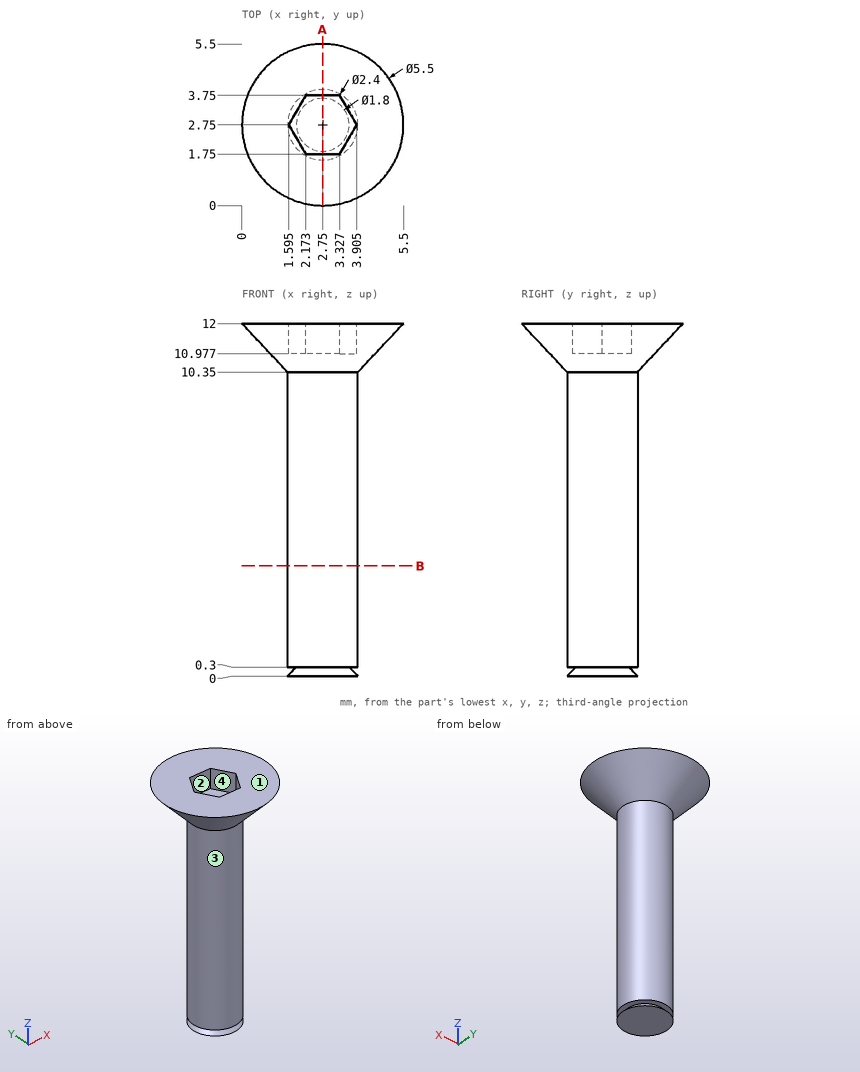
Geometry check sheet. Reference: drawing and pictorial views, mm from the part's lowest x, y, z. Give positions to 0.01 mm unless a question says otherwise; leave off trailing zeros. Write each loop counter-clockwise with the first axis right and the second up, starting at its lowest first coordinate (ties: lowest second). Pieces come first, ordered by that corner, then holes. Notation, with made-up numbers: (-12.75, 31.5) -> (5.25, 31.5) arc R22 cw to (5.25, 67.5) -> close; hole circle Ø1 at (-22, -38.5). An arc over 180 degrees is marked (long way). One line per item, written item: value. Start each with the question number.
Item 1: Material ranges on probe 1 along Z at (x, y) = (3.5, 2.6); probe 2 along Y at (x, z) = (2.8, 8.25); probe 3 along X at (y, z) = (3.1, 11.25) (1 decimal), recorded low to high. Write a range as from..to.
Item 2: Draft check along X on the marked faces 1, 2, 3 and 4. Enter one of: +X half, -X half, draft (parallel to the pull), parting line (faces both ways), or undercut.
Item 3: Section check B-B on z = 3.75. Record the cut outline in (x, y).
Item 4: Section check A-A on x = 2.75. Record the cut outline in (y, z).
Item 5: Gauge pin test, flat ends, axial feed: pin 1 (0.8 mm diameter, centred on x = 2.5, z = 11.5, fed in from +Y) (1 decimal); pin 2 (2 mm diameter, centred on x = 4.5, z = 4.5, fed in from +Y); pin 3 (0.7 mm diameter, centred on x = 2.5, y = 2.5, fed in from -Z); pin 4 (1 mm diameter, centred on x = 3, y = 2.5, fed in from +Z). Record the tip position at first contact, or that the pin passes through.
Results list:
1. probe 1: 0..10.98
1. probe 2: 1.55..3.95
1. probe 3: 0.7..1.8, 3.7..4.8
2. face 1: draft
2. face 2: undercut
2. face 3: parting line
2. face 4: undercut
3. outline: circle Ø2.4 at (2.75, 2.75)
4. outline: (0, 12) -> (1.55, 10.35) -> (1.55, 0.3) -> (1.85, 0.3) -> (1.55, 0) -> (3.95, 0) -> (3.65, 0.3) -> (3.95, 0.3) -> (3.95, 10.35) -> (5.5, 12) -> (3.75, 12) -> (3.75, 10.98) -> (1.75, 10.98) -> (1.75, 12) -> close
5. pin 1: y = 5.4
5. pin 2: y = 3.69
5. pin 3: z = 0
5. pin 4: z = 10.98
